The listing builds one solid part. Answer for the finished solid, in the listing's coordinates (mm). A direction names the side the tool comes from. Coordinates: 2 decimals unless noted, no trailing zeros. Order: outer loops, then holes, each group sorted by start corner. A loop starts at its lowest first (then second) coordinate and runs counter-clockwise, first axis right, second up.
Autodesk Inventor part; units mm, degrees
ref_plane "YZ Plane" through (0, 0, 0) normal (1, 0, 0) x (0, 1, 0)
ref_plane "XZ Plane" through (0, 0, 0) normal (0, 1, 0) x (-1, 0, 0)
ref_plane "XY Plane" through (0, 0, 0) normal (0, 0, 1) x (1, 0, 0)
sketch "Sketch1" plane through (0, 0, 0) normal (0, 0, 1) x (1, 0, 0)
  line L0 (3.175, 0) -> (22.225, 0)
  line L1 (25.4, 3.175) -> (25.4, 22.225)
  line L2 (22.225, 25.4) -> (3.175, 25.4)
  line L3 (0, 22.225) -> (0, 3.175)
  arc A0 (3.175, 25.4) -> (0, 22.225) centre (3.175, 22.225) ccw
  arc A1 (25.4, 22.225) -> (22.225, 25.4) centre (22.225, 22.225) ccw
  arc A2 (22.225, 0) -> (25.4, 3.175) centre (22.225, 3.175) ccw
  arc A3 (0, 3.175) -> (3.175, 0) centre (3.175, 3.175) ccw
  line L4 (6.35, 3.175) -> (19.05, 3.175)
  line L5 (22.225, 6.35) -> (22.225, 19.05)
  line L6 (19.05, 22.225) -> (6.35, 22.225)
  line L7 (3.175, 19.05) -> (3.175, 6.35)
  arc A4 (6.35, 22.225) -> (3.175, 19.05) centre (6.35, 19.05) ccw
  arc A5 (19.05, 3.175) -> (22.225, 6.35) centre (19.05, 6.35) ccw
  arc A6 (22.225, 19.05) -> (19.05, 22.225) centre (19.05, 19.05) ccw
  arc A7 (3.175, 6.35) -> (6.35, 3.175) centre (6.35, 6.35) ccw
  point P0 (0, 0)
  point P1 (25.4, 25.4)
  point P2 (25.4, 0)
  point P3 (0, 25.4)
  dimension "d0" = 25.4
  dimension "d1" = 25.4
  dimension "d2" = 3.175
  dimension "d3" = 3.175
extrude "Extrusion1" add sketch "Sketch1" along normal blind 438.15
properties part number "FrontHorizTop"
1) Section C-C (z = 103) is taken. Give the vertices of the cut face in (x, y) (3 decimals), then the cut area to 3 significant figures.
2) Determine the mould class of faces 1 (the face through (0, 13, 216)), 2 (the face through (22.225, 13, 216)), 3 (the face through (3.175, 13, 216)), 4 (the face through (1, 13, 0)) for opening direction X: released by +X, released by -X, zero draft, split by the parting line, or undercut.
3) Consider L1, parallel to Y at x = 15.5, z = 181 (3 decimals); L2, parallel to X at y = 19.75, z = 326.5. Determine where each line is inside the solid, lowest interval first.
4) Section A-A (x = 14.25) is taken. Give the vertices of the cut face in (y, z) (3 decimals).
5) A tool of negligible diameter and unlimited length cuts with its end or side. For faces 5 (the face through (13, 0, 216)), 6 (the face through (13, 3.175, 216)), from which of +Z, -Z, +X, -X, +Y, -Y can it reach the whole face along a straight path? Write none if from no direction.
Filled sheet:
1. outline: (0, 3.175) arc R3.175 ccw to (3.175, 0) - (22.225, 0) arc R3.175 ccw to (25.4, 3.175) - (25.4, 22.225) arc R3.175 ccw to (22.225, 25.4) - (3.175, 25.4) arc R3.175 ccw to (0, 22.225) - close; hole (3.175, 6.35) arc R3.175 ccw to (6.35, 3.175) - (19.05, 3.175) arc R3.175 ccw to (22.225, 6.35) - (22.225, 19.05) arc R3.175 ccw to (19.05, 22.225) - (6.35, 22.225) arc R3.175 ccw to (3.175, 19.05) - close
1. area: 282 mm2
2. face 1: released by -X
2. face 2: undercut
2. face 3: undercut
2. face 4: zero draft
3. L1: y = 0 to 3.175, 22.225 to 25.4
3. L2: x = 0 to 3.25, 22.15 to 25.4
4. outline: (0, 0) - (3.175, 0) - (3.175, 438.15) - (0, 438.15) - close; (22.225, 0) - (25.4, 0) - (25.4, 438.15) - (22.225, 438.15) - close
5. face 5: +Z, -Z, +X, -X, -Y
5. face 6: +Z, -Z
